Verification items for the finished model (mm, model axes). A direction names the side the tool comes from. Round coordinates to 2 decimals unless told otherwise and drop trailing zeros. Write each loop counter-clockwise with the first axis right and the second up, starting at its lowest first coordinate (ties: lowest second). Pieces come first, ordered by that corner, then holes. Notation, with made-up numbers: M 56,-39.5 L 106,-39.5 A8 cw 106,-26.5 Z; hole C 74.5,61.5 d5. An arc over 180 degrees is marked long. Write each question's results on one line, items separated by ' | '.
from build123d import *

# Parameters (mm, degrees)
SKETCH_1_W      = 20
SKETCH_1_H      = 20
EXTRUDE_1_DEPTH = 1.5
SKETCH_2_R      = 2.5
EXTRUDE_2_DEPTH = 5
FILLET_1_R      = 1.5
FILLET_2_R      = 0.5


with BuildPart() as part:
    # 草图1 → 凸台-拉伸1 (new body)
    with BuildSketch(Plane(origin=(0, 0, 0), x_dir=(1, 0, 0), z_dir=(0, 1, 0))):
        Rectangle(SKETCH_1_W, SKETCH_1_H)
    extrude(amount=EXTRUDE_1_DEPTH)

    # 草图2 → 凸台-拉伸2 (add)
    with BuildSketch(Plane(origin=(0, 1.5, 0), x_dir=(1, 0, 0), z_dir=(0, 1, 0))):
        with Locations(Location((0, 0, 0), (0, 0, 270))):
            Circle(SKETCH_2_R)
    extrude(amount=EXTRUDE_2_DEPTH)

    # 圆角1
    fillet_1_edges = [part.edges().sort_by_distance(p)[0] for p in [
        (0, 0, 10),
        (10, 0, 0),
        (0, 0, -10),
        (-10, 0, 0),
    ]]
    fillet(fillet_1_edges, radius=FILLET_1_R - 0.0001)  # a hair under: the kernel refuses the full size

    # 圆角2
    fillet_2_edges = [part.edges().sort_by_distance(p)[0] for p in [
        (0, 6.5, -2.5),
    ]]
    fillet(fillet_2_edges, radius=FILLET_2_R)


solid = part.part
1) Sectioned sample at C-C, the plane y = 4.5. Record the cut outline in (x, z).
Calculated:
outline: C 0,0 d5
2) Access from +Z, -Z, +X, -X, +Y, -Y to the whole of each face (thin tool, end or side, straight path). Record for faces 1 (the flat face through (-2, 1.5, 2)), 2 (the flat face through (0, 6.5, 0)).
Calculated:
face 1: +Y | face 2: +Z, -Z, +X, -X, +Y
3) Depth check by flat-ended pin: P1, Ø1, axis at y = 2.5, z = 6.5, coming from the -X side; P2, Ø3, axis at y = 4.5, z = -2.5, coming from the -X side; P3, Ø1.5, axis at x = 4.5, z = -4.5, coming from the +Y side. Enter the tip coordinate at first touch or a pass-through.
Calculated:
P1: passes through | P2: stops at x = -2.29 | P3: stops at y = 1.5
4) Material ranges on line 1 (Y direction, x = 6, z = 3.25); line 2 (X direction, y = 3.75, z = 1.5); line 3 (Z direction, x = 4.25, y = 1), recorded low to high. Write a range as [from, to].
Calculated:
line 1: y = [0, 1.5] | line 2: x = [-2, 2] | line 3: z = [-9.91, 9.91]
